Can you work these out from the model? Positions are in its coordinate system, mm. Face numbers are marked on the shaded views. A direction names the side the tool comes from. Give positions to 0.01 mm unless a question says otherwise; leave off trailing zeros. Order: outer loops, then holes, each group sorted by start corner. A loop starts at its lowest first (then second) coordinate and runs counter-clockwise, first axis right, second up. Notation, with made-up numbers: (84, 44) - (125, 44) arc R15 ccw to (125, 52) - close; hole circle Ø8 at (16, 77). An arc over 180 degrees is marked (long way). Use one line per item in the form item = value. Start each with the question number.
1) Suppose I cut it at B-B, the plane z = 0. Write out the boundary of the cut face in (x, y), and give its area (3 significant figures).
2) Which directions (+Z, -Z, +X, -X, +Y, -Y) give clear straight access to the entire face, cutting with the end or side of a thin tool? Please do the marked faces 1 and 2.
3) We'd pull the mould along Z, two halves only. Please class the marked faces 3, 4 and 5: released by +Z, released by -Z, zero draft, split by the parting line, or undercut.
4) Please list where these lines run through material, in increasing order: probe 1 along Z at (x, y) = (4.25, -5); probe 2 along X at (y, z) = (0.25, 8.5); probe 3 along Z at (x, y) = (2.75, -3.5).
5) Suppose I cut it at C-C, the plane x = 4. Write out the boundary of the cut face in (y, z), and give its area (3 significant figures).
6) For pin 1 (2 mm diameter, centred on y = 1, z = 7, fed in from -X); pin 2 (4 mm diameter, centred on y = 1.5, z = -8, fed in from +X); pin 3 (6 mm diameter, centred on x = 1, y = 2, fed in from +Z), each with a flat end and sliding along its axis, tell me the tip position at first contact or that it passes through.
7) Suppose I cut it at A-A, the plane y = -5. Write out the boundary of the cut face in (x, z).
```python
from build123d import *

# Parameters (mm, degrees)
SFAZOWANIE1_SIZE = 0.5


with BuildPart() as part:
    # Szkic1 → Obrót1 (revolve)
    with BuildSketch(Plane.XY):
        with BuildLine():
            Line((-7, 0), (7, 0))
            Line((7, 0), (7, 1.45))
            ThreePointArc((7, 1.45), (6.170128128, 2.247897549), (5.25, 2.939773297))
            Line((5.25, 2.939773297), (5.25, 6))
            Line((5.25, 6), (-5.25, 6))
            Line((-5.25, 6), (-5.25, 2.939773297))
            ThreePointArc((-5.25, 2.939773297), (-6.170128128, 2.247897549), (-7, 1.45))
            Line((-7, 1.45), (-7, 0))
        make_face()
    revolve(axis=Axis((-7.6504069, -5, 0), (1, 0, 0)))

    # Sfazowanie1
    sfazowanie1_edges = [part.edges().sort_by_distance(p)[0] for p in [
        (-5.25, -16, 0),
        (5.25, -16, 0),
    ]]
    chamfer(sfazowanie1_edges, length=SFAZOWANIE1_SIZE)


solid = part.part
```
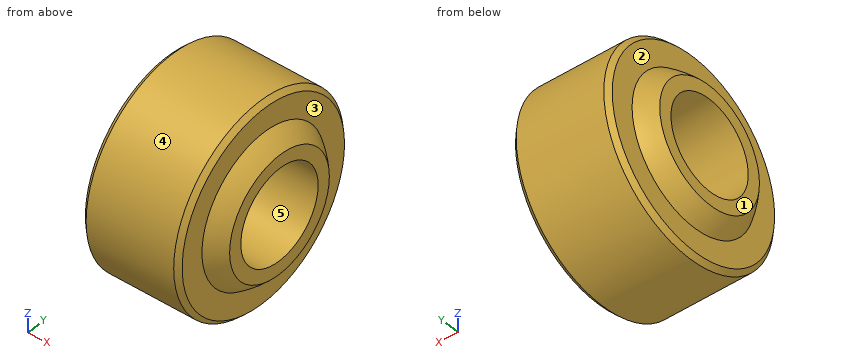
Result sheet:
q1.outline = (-7, -11.45) arc R9.52 ccw to (-5.25, -12.94) - (-5.25, -15.5) - (-4.75, -16) - (4.75, -16) - (5.25, -15.5) - (5.25, -12.94) arc R9.52 ccw to (7, -11.45) - (7, -10) - (-7, -10) - close; (-7, 0) - (7, 0) - (7, 1.45) arc R9.52 ccw to (5.25, 2.94) - (5.25, 5.5) - (4.75, 6) - (-4.75, 6) - (-5.25, 5.5) - (-5.25, 2.94) arc R9.52 ccw to (-7, 1.45) - close
q1.area = 141 mm²
q2.face_1 = +Z, -Z, -X, +Y, -Y
q2.face_2 = -X
q3.face_3 = zero draft
q3.face_4 = split by the parting line
q3.face_5 = undercut
q4.probe_1 = -11 to -5, 5 to 11
q4.probe_2 = -5.25 to 5.25
q4.probe_3 = -10.9 to -4.77, 4.77 to 10.9
q5.outline = circle Ø22 at (-5, 0); hole circle Ø10 at (-5, 0)
q5.area = 302 mm²
q6.pin_1 = -5.25
q6.pin_2 = 5.25
q6.pin_3 = 10.25
q7.outline = (-7, -6.45) arc R9.52 ccw to (-5.25, -7.94) - (-5.25, -10.5) - (-4.75, -11) - (4.75, -11) - (5.25, -10.5) - (5.25, -7.94) arc R9.52 ccw to (7, -6.45) - (7, -5) - (-7, -5) - close; (-7, 5) - (7, 5) - (7, 6.45) arc R9.52 ccw to (5.25, 7.94) - (5.25, 10.5) - (4.75, 11) - (-4.75, 11) - (-5.25, 10.5) - (-5.25, 7.94) arc R9.52 ccw to (-7, 6.45) - close
